Can you work these out from the model? Positions are in its coordinate system, mm. A direction names the side the tool comes from. Give positions to 0.01 mm unless a question says otherwise; leave off trailing zeros. Order: outer loops, then holes, each group sorted by start corner. A loop starts at its lowest first (then second) coordinate and runs counter-clockwise, first axis right, second up. Notation, with made-up numbers: (78, 26.25) - (129, 26.25) arc R14 ccw to (129, 42.25) - close; hole circle Ø7 at (27, 36). An arc over 180 degrees is marked (long way). One line per question, with ' | ' between items.
```python
from build123d import *

# Parameters (mm, degrees)
SKETCH3_R           = 3.81
BOSS_EXTRUDE1_DEPTH = 12.827
CHAMFER1_SIZE       = 0.381


with BuildPart() as part:
    # Sketch1 → Revolve1 (revolve)
    with BuildSketch(Plane.XY):
        Polygon((-12.8778, 10.668), (-12.8778, 3.81), (0.2032, 3.81), (0.2032, 2.38125), (-24.036969082, 2.38125), (-28.412119082, 6.7564), (-28.412119082, 7.7724), (-15.712119082, 7.7724), (-15.712119082, 10.668), align=None)
    revolve(axis=Axis((-22.598839253, 0, 0), (1, 0, 0)))

    # Sketch3 → Boss-Extrude1 (add)
    with BuildSketch(Plane(origin=(-12.8778, 0, 0), x_dir=(0, 0, -1), z_dir=(1, 0, 0))):
        Polygon((-4.7879, 2.764295354), (-4.7879, -2.764295354), (0, -5.528590708), (4.7879, -2.764295354), (4.7879, 2.764295354), (0, 5.528590708), align=None)
        Circle(SKETCH3_R, mode=Mode.SUBTRACT)
    extrude(amount=BOSS_EXTRUDE1_DEPTH)

    # Chamfer1
    chamfer1_edges = [part.edges().sort_by_distance(p)[0] for p in [
        (-0.0508, 4.146443031, 2.39395),
        (-0.0508, 0, 4.7879),
        (-0.0508, -4.146443031, 2.39395),
        (-0.0508, -4.146443031, -2.39395),
        (-0.0508, 0, -4.7879),
        (-0.0508, 4.146443031, -2.39395),
    ]]
    chamfer(chamfer1_edges, length=CHAMFER1_SIZE)


solid = part.part
```
(1) Imagine slicing it at D-D (z = 9.25). List the corners of the cut face in (x, y) for me, and give its area (3 significant figures).
Answer below:
outline: (-15.71, -5.31) - (-12.88, -5.31) - (-12.88, 5.31) - (-15.71, 5.31) - close | area: 30.1 mm^2
(2) Imagine slicing it at B-B (x = -5.75). List the corners of the cut face in (y, z) for me.
Answer below:
outline: (-5.53, 0) - (-2.76, -4.79) - (2.76, -4.79) - (5.53, 0) - (2.76, 4.79) - (-2.76, 4.79) - close; hole circle Ø4.76 at (0, 0)
(3) Imagine slicing it at A-A (y = 0). List the corners of the cut face in (x, z) for me, and give its area (3 significant figures).
Answer below:
outline: (-28.41, -7.77) - (-15.71, -7.77) - (-15.71, -10.67) - (-12.88, -10.67) - (-12.88, -4.79) - (-0.43, -4.79) - (-0.05, -4.41) - (-0.05, -3.81) - (0.2, -3.81) - (0.2, -2.38) - (-24.04, -2.38) - (-28.41, -6.76) - close; (-28.41, 6.76) - (-24.04, 2.38) - (0.2, 2.38) - (0.2, 3.81) - (-0.05, 3.81) - (-0.05, 4.41) - (-0.43, 4.79) - (-12.88, 4.79) - (-12.88, 10.67) - (-15.71, 10.67) - (-15.71, 7.77) - (-28.41, 7.77) - close | area: 227 mm^2
(4) Will these pins go through, and if not, where does the flat tip stop? pin 1 (12 mm diameter, centred on x = -4, y = -1, fed in from +Z); pin 2 (3 mm diameter, centred on x = -5.5, y = 1, fed in from -Z); pin 3 (1.5 mm diameter, centred on y = -2, z = -3.5, fed in from -X).
Answer below:
pin 1: z = 4.79 | pin 2: z = -4.79 | pin 3: x = -26.44
(5) If I drill on line 1 (Z direction, x = -12.25, y = 0); line 2 (Z direction, x = -16, y = 0); line 3 (X direction, y = -7.25, z = 7), over which ranges is the centre line in solid material (lowest first)?
Answer below:
line 1: -4.79 to -2.38, 2.38 to 4.79 | line 2: -7.77 to -2.38, 2.38 to 7.77 | line 3: -15.71 to -12.88
(6) Imagine slicing it at C-C (x = -19.5). List the corners of the cut face in (y, z) for me.
Answer below:
outline: circle Ø15.54 at (0, 0); hole circle Ø4.76 at (0, 0)
(7) If we mould it in two halves opening along Z, with no side actions, what happens to faces 1 (the face through (-0.244, 4.003, 2.267)), 2 (the face through (-24.31, -0.58, -2.59)), 3 (the face through (-6.742, -4.166, -2.36)), 4 (the face through (-12.09, -1.89, -1.45))? For each: released by +Z, released by -Z, zero draft, split by the parting line, or undercut.
Answer below:
face 1: released by +Z | face 2: undercut | face 3: released by -Z | face 4: undercut
(8) On a 3-axis mill with a long thin cutter (end or side, diameter ignored), from which of +Z, -Z, +X, -X, +Y, -Y can I reach the whole of each face in a straight line? I mean faces 5 (the face through (-7, 0, -4.788)), 6 (the face through (-6.742, 4.166, 2.36)), 7 (the face through (-6.742, -4.127, 2.427)), 8 (the face through (-6.742, 4.127, -2.427)), 9 (the face through (-0.051, -4, 1)). Say none if no direction works.
Answer below:
face 5: -Z, +X, +Y, -Y | face 6: +Z, +X, +Y | face 7: +Z, +X, -Y | face 8: -Z, +X, +Y | face 9: +X
